from build123d import *

# Parameters (mm, degrees)
EXTRUDE_1_DEPTH          = 3
CUT_EXTRUDE_1_DEPTH      = 55.863466897
CUT_EXTRUDE_1_DEPTH_BACK = 55.863466897
SKETCH_2_W               = 16
SKETCH_2_H               = 20
FILLET_1_R               = 2
SKETCH_3_W               = 28
SKETCH_3_H               = 23
CUT_EXTRUDE_2_DEPTH      = 10
FILLET_2_R               = 3


with BuildPart() as part:
    # 草图1 → 凸台-拉伸1 (new body)
    with BuildSketch(Plane(origin=(0, 0, 0), x_dir=(1, 0, 0), z_dir=(0, 1, 0))):
        Polygon((20, 48), (16, 48), (16, 51), (6, 51), (6, 48), (-6, 48), (-6, 51), (-16, 51), (-16, 48), (-20, 48), (-20, -18), (20, -18), align=None)
        with BuildLine():
            Line((15.3, 6), (15.3, -2))
            ThreePointArc((15.3, -2), (16.007106781, -3.707106781), (14.3, -3))
            Line((14.3, -3), (13, -3))
            ThreePointArc((13, -3), (11.292893219, -3.707106781), (12, -2))
            Line((12, -2), (12, 6))
            ThreePointArc((12, 6), (11.292893219, 7.707106781), (13, 7))
            Line((13, 7), (14.3, 7))
            ThreePointArc((14.3, 7), (16.007106781, 7.707106781), (15.3, 6))
        make_face(mode=Mode.SUBTRACT)
        with BuildLine():
            Line((-12, 6), (-12, -2))
            ThreePointArc((-12, -2), (-11.292893219, -3.707106781), (-13, -3))
            Line((-13, -3), (-14.3, -3))
            ThreePointArc((-14.3, -3), (-16.007106781, -3.707106781), (-15.3, -2))
            Line((-15.3, -2), (-15.3, 6))
            ThreePointArc((-15.3, 6), (-16.007106781, 7.707106781), (-14.3, 7))
            Line((-14.3, 7), (-13, 7))
            ThreePointArc((-13, 7), (-11.292893219, 7.707106781), (-12, 6))
        make_face(mode=Mode.SUBTRACT)
        with BuildLine():
            Line((-7.65, -12), (-7.65, -10.7))
            ThreePointArc((-7.65, -10.7), (-8.357106781, -8.992893219), (-6.65, -9.7))
            Line((-6.65, -9.7), (6.65, -9.7))
            ThreePointArc((6.65, -9.7), (8.357106781, -8.992893219), (7.65, -10.7))
            Line((7.65, -10.7), (7.65, -12))
            ThreePointArc((7.65, -12), (8.357106781, -13.707106781), (6.65, -13))
            Line((6.65, -13), (-6.65, -13))
            ThreePointArc((-6.65, -13), (-8.357106781, -13.707106781), (-7.65, -12))
        make_face(mode=Mode.SUBTRACT)
    extrude(amount=EXTRUDE_1_DEPTH)

    # 草图2 → 切除-拉伸1 (cut, two sides: drawn at the far end of the back side and taken through both)
    with BuildSketch(Plane(origin=(0, 3, 0), x_dir=(1, 0, 0), z_dir=(0, 1, 0)).offset(-CUT_EXTRUDE_1_DEPTH_BACK)):
        with Locations((0, 4)):
            Rectangle(SKETCH_2_W, SKETCH_2_H)
    extrude(amount=CUT_EXTRUDE_1_DEPTH + CUT_EXTRUDE_1_DEPTH_BACK, mode=Mode.SUBTRACT)

    # 圆角1
    fillet_1_edges = [part.edges().sort_by_distance(p)[0] for p in [
        (8, 1.5, -14),
        (8, 1.5, 6),
        (-8, 1.5, 6),
        (-8, 1.5, -14),
    ]]
    fillet(fillet_1_edges, radius=FILLET_1_R)

    # 草图3 → 切除-拉伸2 (cut)
    with BuildSketch(Plane(origin=(0, 3, 0), x_dir=(1, 0, 0), z_dir=(0, 1, 0))):
        with Locations((0, 31.5)):
            Rectangle(SKETCH_3_W, SKETCH_3_H)
    extrude(amount=-CUT_EXTRUDE_2_DEPTH, mode=Mode.SUBTRACT)

    # 圆角2
    fillet_2_edges = [part.edges().sort_by_distance(p)[0] for p in [
        (14, 1.5, -43),
        (14, 1.5, -20),
        (-14, 1.5, -20),
        (-14, 1.5, -43),
    ]]
    fillet(fillet_2_edges, radius=FILLET_2_R)


solid = part.part
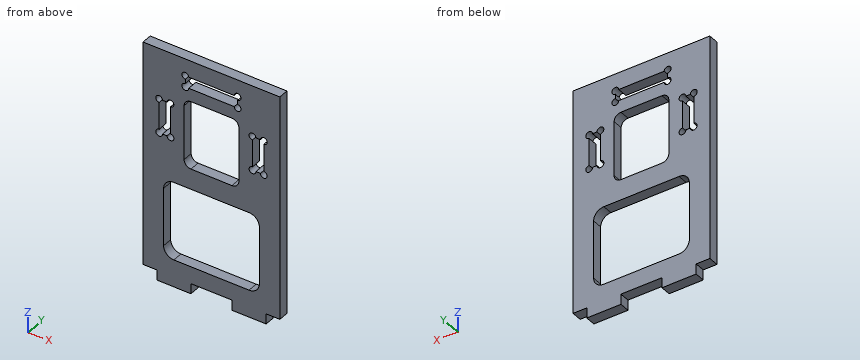
Model file for the job. Use its own axes, mm. Round coordinates to 2 decimals unless told otherwise and drop trailing zeros. Loops run counter-clockwise (first coordinate to the right, second up) from the corner with the lowest first, then second, coordinate; pieces in that order, holes last.
1. Band-saw the part on A-A, the plane z = -5. List the corners of the cut face in (x, y).
Check values:
outline: (-20, 0) - (-15.3, 0) - (-15.3, 3) - (-20, 3) - close; (-12, 0) - (-8, 0) - (-8, 3) - (-12, 3) - close; (8, 0) - (12, 0) - (12, 3) - (8, 3) - close; (15.3, 0) - (20, 0) - (20, 3) - (15.3, 3) - close
2. Drop flat-ended pins along their axis: P1, Ø0.9, axis at x = 0.5, y = 1, coming from the -Z side; P2, Ø1.6, axis at x = -7.65, z = 13, coming from the -Y side; P3, Ø0.9, axis at y = 1, z = -49, coming from the -X side. Give the stop position or say it passes through.
Check values:
P1: stops at z = -48
P2: passes through
P3: stops at x = -16
3. Band-saw the part on C-C, the plane z = -24. List the corners of the cut face in (x, y).
Check values:
outline: (-20, 0) - (-14, 0) - (-14, 3) - (-20, 3) - close; (14, 0) - (20, 0) - (20, 3) - (14, 3) - close
4. Band-saw the part on D-D, the plane y = 0.8. Count the separate pieces of the cut face and the enclosed holes in it, and give its area (3 significant figures).
Check values:
separate pieces: 1
enclosed holes: 5
area: 1,600 mm2
5. Wall check: probe 1 along Z at (x, y) = (5, 0.2); probe 2 along X at (y, z) = (0.25, -5); probe 3 along X at (y, z) = (2.6, -26.5). Give the ranges that are in metal, low to high.
Check values:
probe 1: z = -48 to -43, -20 to -14, 6 to 9.7, 13 to 18
probe 2: x = -20 to -15.3, -12 to -8, 8 to 12, 15.3 to 20
probe 3: x = -20 to -14, 14 to 20
6. Band-saw the part on B-B, the plane x = 0.5. List the corners of the cut face in (y, z).
Check values:
outline: (0, -48) - (3, -48) - (3, -43) - (0, -43) - close; (0, -20) - (3, -20) - (3, -14) - (0, -14) - close; (0, 6) - (3, 6) - (3, 9.7) - (0, 9.7) - close; (0, 13) - (3, 13) - (3, 18) - (0, 18) - close
